from build123d import *

# Parameters (mm, degrees)
F1_R        = 4.5
F1_R_2      = 9
F2_DEPTH    = 5
F3_R        = 7
F4_DEPTH    = 2
F6_S5_R     = 7
F6_T6_DEPTH = 12
F8_DEPTH    = 25.002
F11_REACH   = 49.0720678119


# Not quite as in the source:
# - a fillet or chamfer that OpenCascade refuses, or shapes differently, is made with other operations: its cross-section is extruded or revolved along the edge and cut away or added


with BuildPart() as f2:
    # F1 (on Front) → F2 (new body)
    with BuildSketch(Plane.XZ):
        with BuildLine():
            ThreePointArc((-17.5, 21.3840905163), (-19.5315060063, 20.829810085), (-21, 19.3205821894))
            Line((-21, 19.3205821894), (-21, 0.2360721162))
            Line((-21, 0.2360721162), (-19.0729714288, -3.6179094837))
            Line((-19.0729714288, -3.6179094837), (19.0729714288, -3.6179094837))
            Line((19.0729714288, -3.6179094837), (21, 0.2360721162))
            Line((21, 0.2360721162), (21, 19.3205821894))
            ThreePointArc((21, 19.3205821894), (19.5315060063, 20.829810085), (17.5, 21.3840905163))
            Line((17.5, 21.3840905163), (-17.5, 21.3840905163))
        make_face()
        with Locations((-12.3, 13)):
            Circle(F1_R, mode=Mode.SUBTRACT)
        with Locations((10.94, 11.55)):
            Circle(F1_R_2, mode=Mode.SUBTRACT)
    extrude(amount=F2_DEPTH)

    # F3 (on face) → F4 (cut)
    with BuildSketch(Plane.XZ.offset(5)):
        with Locations((-12.3, 13)):
            Circle(F3_R)
    extrude(amount=-F4_DEPTH, mode=Mode.SUBTRACT)

    # F5: chamfer of 2 on 1 edges, made by hand

    # F5_s1 → F5_t2 (revolve, cut)
    with BuildSketch(Plane.XY.offset(11.55)):
        Polygon((21.94, -5), (19.94, -3), (19.94, -5), align=None)
    revolve(axis=Axis((10.94, -5, 11.55), (0, -1, 0)), mode=Mode.SUBTRACT)

    # F6: chamfer of 3 on 1 edges, made by hand


with BuildPart() as f6_tool2:
    # F6_s3 → F6_t4 (revolve)
    with BuildSketch(Plane.XY.offset(13)):
        Polygon((-7.8, 0), (-4.8, -3), (-7.8, -3), align=None)
    revolve(axis=Axis((-12.3, -3, 13), (0, 1, 0)))

    # F6_s5 → F6_t6 (intersect, symmetric)
    with BuildSketch(Plane.XZ.offset(1.5)):
        with Locations((-12.3, 13)):
            Circle(F6_S5_R)
    extrude(amount=F6_T6_DEPTH, both=True, mode=Mode.INTERSECT)


with BuildPart() as f2_1:
    add(f2.part)

    # F6_t1: cut F6_tool2
    add(f6_tool2.part, mode=Mode.SUBTRACT)

    # F7 (on face) → F8 (cut, through all)
    with BuildSketch(Plane(origin=(0, 0, -3.6179094837), x_dir=(1, 0, 0), z_dir=(0, 0, -1))):
        Polygon((-21, 5), (-21, 0), (-12.3, 5), align=None)
        Polygon((21, 5), (10.94, 5), (21, 0), align=None)
    extrude(amount=-F8_DEPTH, mode=Mode.SUBTRACT)

    f11_end = Plane(origin=(-17.3406659547, -2.1030655433, 7.002775246), x_dir=(-0.867013944, 0.4982838759, 0), z_dir=(-0.4982838759, -0.867013944, 0))
    # F10 (on offset) → F11 (cut, up to a plane its end follows)
    with BuildSketch(Plane.YZ.offset(21)):
        Polygon((-5, -3.6179094837), (0, -3.6179094837), (-5, 1.3820905163), align=None)
    f11_long = extrude(amount=-F11_REACH, mode=Mode.PRIVATE)
    add(split(f11_long, bisect_by=f11_end, keep=Keep.BOTTOM, mode=Mode.PRIVATE), mode=Mode.SUBTRACT)


solid = f2_1.part
Model file for the job. Use its own axes, mm. Give positions to 0.01 mm unless a question says otherwise; leave off trailing zeros. Loops run counter-clockwise (first coordinate to the right, second up) from the corner with the lowest first, then second, coordinate; pieces in that order, holes last. Notation, with made-up numbers: (82, 78) -> (86, 78) arc R24 ccw to (86, 97) -> close; hole circle Ø11 at (-14.75, 53.5). An arc over 180 degrees is marked (long way). Use a Markdown table: item, result. Add a question column.
(1) Slice it at B-B on z = 17. Give the number of separate pieces and of enclosed holes in the cut face, and give its area (3 significant figures).
(2) Mould opens along Z. For faces 1 (the flat face through (19.39, -0.8, 6.4)), 2 (the flat face through (0, -2, 21.384)), 3 (the cylindrical face through (-5.303, -3.768, 12.78)) say: +Z half, -Z half, draft (parallel to the pull), parting line (faces both ways), or undercut.
(3) Wall check: line 1 along X through (y, z) = (-0.6, 15.5); line 2 along Z through (x, y) = (10.94, -0.7); line 3 along Z through (x, y) = (7.5, -1.25). Give the ranges that are in metal, low to high.
(4) Slice it at A-A on x = 17. List the corners of the cut face in (y, z), and give its area (3 significant figures).
(5) Slice it at C-C on x = 10.94. List the corners of the cut face in (y, z).
(6) Drop a flat-ended pin along its axis: pin 1 Ø1.5 at (y, z) = (-4, 18) entering from -X. Give the stop position or say it passes through.
Filled sheet:
| question | item | result |
|---|---|---|
| 1 | separate pieces | 3 |
| 1 | enclosed holes | 0 |
| 1 | area | 62.0 mm2 |
| 2 | face 1 | draft |
| 2 | face 2 | +Z half |
| 2 | face 3 | undercut |
| 3 | line 1 | -19.96 to -16.75, -7.85 to 2.85, 19.03 to 19.79 |
| 3 | line 2 | -2.92 to 2.55, 20.55 to 21.38 |
| 3 | line 3 | -2.37 to 3.23, 19.87 to 21.38 |
| 4 | outline | (-1.99, -1.63) -> (0, -3.62) -> (0, 4.9) -> (-1.99, 4.9) -> close; (-1.99, 18.2) -> (0, 18.2) -> (0, 21.38) -> (-1.99, 21.38) -> close |
| 4 | area | 21.3 mm2 |
| 5 | outline | (-4.58, 0.97) -> (0, -3.62) -> (0, 2.55) -> (-3, 2.55) -> close; (-3.83, 21.38) -> (-3, 20.55) -> (0, 20.55) -> (0, 21.38) -> close |
| 6 | pin 1 | x = -8.31 |
